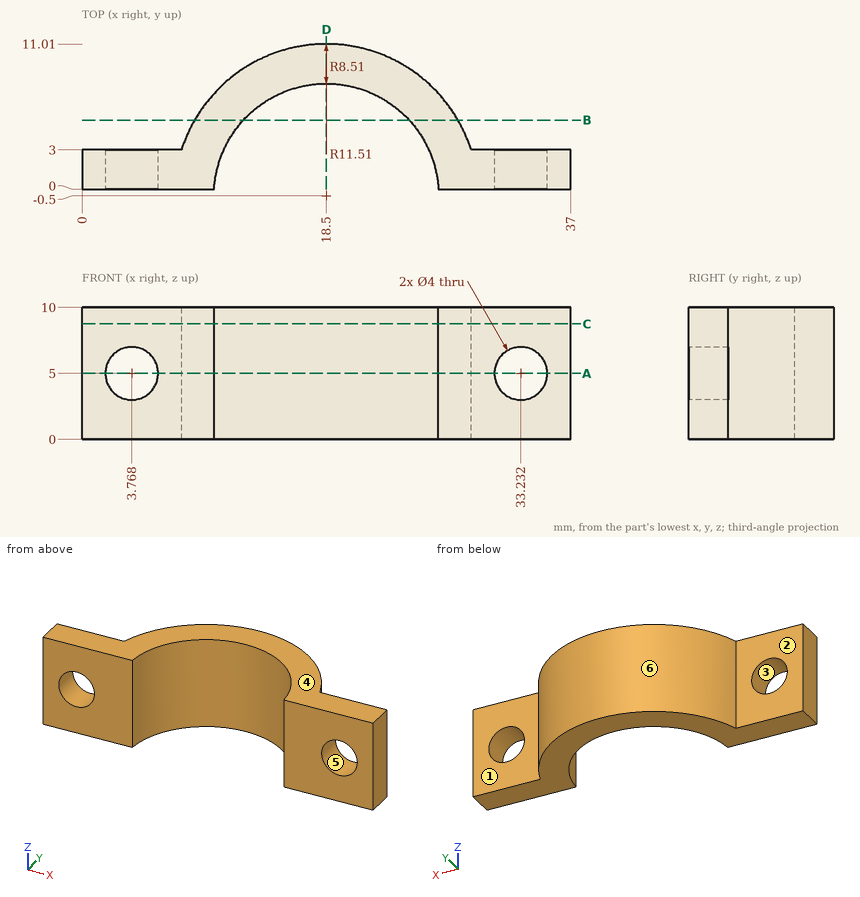
Source: three-view drawing plus pictorial views. Frame: mm from the lowest corner of the part. A direction names the side the tool comes from. Give positions to 0.01 mm unless a question says otherwise; leave off trailing zeros. Order: outer loops, then holes, each group sorted by start corner. A loop starts at its lowest first (then second) coordinate and runs counter-clockwise, first axis right, second up.
1. Section B-B on y = 5.25. Return the cut outline in (x, z).
Derived:
outline: (8.53, 0) - (12.23, 0) - (12.23, 10) - (8.53, 10) - close; (24.77, 0) - (28.47, 0) - (28.47, 10) - (24.77, 10) - close
2. Mould query, pull axis X, two halves, no side actions, for the marked faces 4, 5 and 6. Classes: released by +X, released by -X, zero draft, split by the parting line, or undercut.
Derived:
face 4: zero draft
face 5: undercut
face 6: split by the parting line
3. Section C-C on z = 8.75. Return the cut outline in (x, y) (1 decimal).
Derived:
outline: (0, 0) - (10, 0) arc R8.5 cw to (27, 0) - (37, 0) - (37, 3) - (29.5, 3) arc R11.5 ccw to (7.5, 3) - (0, 3) - close
4. Section D-D on x = 18.5. Return the cut outline in (y, z), and give its area (3 significant figures).
Derived:
outline: (8.01, 0) - (11.01, 0) - (11.01, 10) - (8.01, 10) - close
area: 30.0 mm2
5. Pin query (flat end, axial travel): pin 1 (1 mm diameter, centred on x = 16, z = 2, fed in from +Y) (1 decimal); pin 2 (1.5 mm diameter, centred on x = 15, y = 7.5, fed in from -Z); pin 3 (5 mm diameter, centred on x = 20, z = 3, fed in from -Y); pin 4 (1.5 mm diameter, centred on x = 31, z = 6.5, fed in from +Y). Return the tip coordinate at first contact, or that it passes through.
Derived:
pin 1: stops at y = 10.8
pin 2: stops at z = 0
pin 3: stops at y = 7.01
pin 4: stops at y = 3
6. Material intervals for L1, parallel to Y at x = 3, z = 1.75; L2, parallel to X at y = 3.25, z = 6.75; L3, parallel to X at y = 4.5, z = 7.25 (1 decimal), sorted ascending.
Derived:
L1: y = 0 to 3
L2: x = 7.62 to 10.86, 26.14 to 29.38
L3: x = 8.1 to 11.6, 25.4 to 28.9
7. Reachability of the marked faces 1, 2 and 3 from +Z, -Z, +X, -X, +Y, -Y: full face, straight path, thin tool, end or side. Return the list, or none.
Derived:
face 1: +Z, -Z, +X, +Y
face 2: +Z, -Z, -X, +Y
face 3: +Y, -Y
8. Section A-A on z = 5. Return the cut outline in (x, y) (1 decimal).
Derived:
outline: (0, 0) - (1.8, 0) - (1.8, 3) - (0, 3) - close; (5.8, 0) - (10, 0) arc R8.5 cw to (27, 0) - (31.2, 0) - (31.2, 3) - (29.5, 3) arc R11.5 ccw to (7.5, 3) - (5.8, 3) - close; (35.2, 0) - (37, 0) - (37, 3) - (35.2, 3) - close
